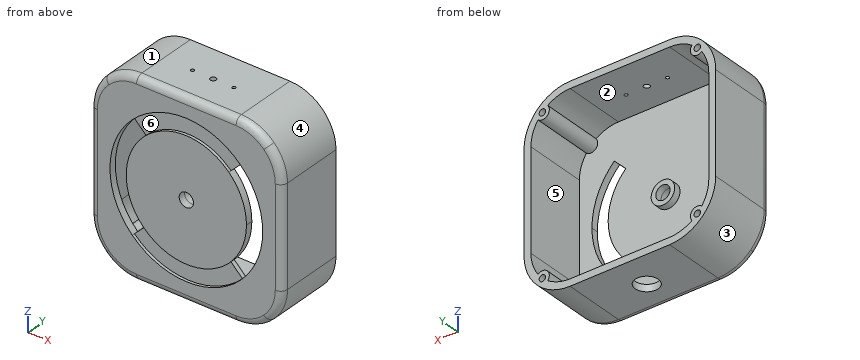
from build123d import *
from build123d.topology import SkipClean

# Parameters (mm, degrees)
SKETCH1_W           = 83.2
SKETCH1_H           = 83.2
BOSS_EXTRUDE1_DEPTH = 30
FILLET1_R           = 20
SHELL2_T            = -3
SKETCH2_R           = 1.25
SKETCH2_R_2         = 0.75
CUT_EXTRUDE1_DEPTH  = 30
SKETCH3_R           = 5
CUT_EXTRUDE2_DEPTH  = 30
SKETCH4_R           = 3.1
CUT_EXTRUDE3_DEPTH  = 30
CUT_EXTRUDE4_DEPTH  = 1.2
SKETCH6_R           = 5.1
SKETCH6_R_2         = 3.1
BOSS_EXTRUDE2_DEPTH = 3
SKETCH7_R           = 3
BOSS_EXTRUDE3_DEPTH = 27
SKETCH9_R           = 1.4
CUT_EXTRUDE5_DEPTH  = 27
FILLET2_R           = 3


with BuildPart() as part:
    # Sketch1 → Boss-Extrude1 (new body)
    with BuildSketch(Plane(origin=(0, 0, 0), x_dir=(1, 0, 0), z_dir=(0, 1, 0))):
        with Locations((-19.461988304, -3.284210526)):
            Rectangle(SKETCH1_W, SKETCH1_H)
    extrude(amount=BOSS_EXTRUDE1_DEPTH)

    # Fillet1
    fillet1_edges = [part.edges().sort_by_distance(p)[0] for p in [
        (-61.061988304, 15, -38.315789474),
        (22.138011696, 15, -38.315789474),
        (22.138011696, 15, 44.884210526),
        (-61.061988304, 15, 44.884210526),
    ]]
    fillet(fillet1_edges, radius=FILLET1_R)

    # Shell2
    shell2_openings = [part.faces().sort_by_distance(p)[0] for p in [
        (-19.461988304, 30, 3.284210526),
    ]]
    offset(amount=SHELL2_T, openings=shell2_openings, kind=Kind.INTERSECTION)

    # Sketch2 → Cut-Extrude1 (cut)
    with BuildSketch(Plane.XY.offset(44.884210526)):
        with Locations((-19.461988304, 15)):
            Circle(SKETCH2_R)
        with Locations((-10.461988304, 15)):
            Circle(SKETCH2_R_2)
        with Locations((-28.461988304, 15)):
            Circle(SKETCH2_R_2)
    extrude(amount=-CUT_EXTRUDE1_DEPTH, mode=Mode.SUBTRACT)

    # Sketch3 → Cut-Extrude2 (cut)
    with BuildSketch(Plane(origin=(0, 0, -38.315789474), x_dir=(-1, 0, 0), z_dir=(0, 0, -1))):
        with Locations((19.461988304, 15)):
            Circle(SKETCH3_R)
    extrude(amount=-CUT_EXTRUDE2_DEPTH, mode=Mode.SUBTRACT)

    # Sketch4 → Cut-Extrude3 (cut)
    with BuildSketch(Plane.XZ):
        with BuildLine():
            ThreePointArc((13.688011696, 3.284210526), (11.164618199, 15.970166309), (3.978601492, 26.724800323))
            Line((3.978601492, 26.724800323), (-1.006501315, 21.739697515))
            ThreePointArc((-1.006501315, 21.739697515), (4.651267494, 13.272248111), (6.638011696, 3.284210526))
            ThreePointArc((6.638011696, 3.284210526), (4.651267494, -6.703827058), (-1.006501315, -15.171276463))
            Line((-1.006501315, -15.171276463), (3.978601492, -20.15637927))
            ThreePointArc((3.978601492, -20.15637927), (11.164618199, -9.401745257), (13.688011696, 3.284210526))
        make_face()
        with BuildLine():
            Line((-37.917475293, 21.739697515), (-42.9025781, 26.724800323))
            ThreePointArc((-42.9025781, 26.724800323), (-52.611988304, 3.284210526), (-42.9025781, -20.15637927))
            Line((-42.9025781, -20.15637927), (-37.917475293, -15.171276463))
            ThreePointArc((-37.917475293, -15.171276463), (-45.561988304, 3.284210526), (-37.917475293, 21.739697515))
        make_face()
        with Locations(Location((-19.461988304, 3.284210526, 0), (0, 0, 270))):
            Circle(SKETCH4_R)
    extrude(amount=-CUT_EXTRUDE3_DEPTH, mode=Mode.SUBTRACT)

    # Sketch5 → Cut-Extrude4 (cut)
    with SkipClean():  # the faces are left unmerged after this step: merging them gives an invalid solid
        with BuildSketch(Plane.XZ):
            with BuildLine():
                Line((-42.9025781, 26.724800323), (-37.917475293, 21.739697515))
                ThreePointArc((-37.917475293, 21.739697515), (-19.461988304, 29.384210526), (-1.006501315, 21.739697515))
                Line((-1.006501315, 21.739697515), (3.978601492, 26.724800323))
                ThreePointArc((3.978601492, 26.724800323), (-19.461988304, 36.434210526), (-42.9025781, 26.724800323))
            make_face()
            with BuildLine():
                Line((-1.006501315, -15.171276463), (3.978601492, -20.15637927))
                ThreePointArc((3.978601492, -20.15637927), (-19.461988304, -29.865789474), (-42.9025781, -20.15637927))
                Line((-42.9025781, -20.15637927), (-37.917475293, -15.171276463))
                ThreePointArc((-37.917475293, -15.171276463), (-19.461988304, -22.815789474), (-1.006501315, -15.171276463))
            make_face()
        extrude(amount=-CUT_EXTRUDE4_DEPTH, mode=Mode.SUBTRACT)

    # Sketch6 → Boss-Extrude2 (add)
    with SkipClean():  # the faces are left unmerged after this step: merging them gives an invalid solid
        with BuildSketch(Plane(origin=(0, 3, 0), x_dir=(1, 0, 0), z_dir=(0, 1, 0))):
            with Locations(Location((-19.461988304, -3.284210526, 0), (0, 0, 270))):
                Circle(SKETCH6_R)
            with Locations(Location((-19.461988304, -3.284210526, 0), (0, 0, 90))):
                Circle(SKETCH6_R_2, mode=Mode.SUBTRACT)
        extrude(amount=BOSS_EXTRUDE2_DEPTH)

    # Sketch7 → Boss-Extrude3 (add)
    with SkipClean():  # the faces are left unmerged after this step: merging them gives an invalid solid
        with BuildSketch(Plane(origin=(0, 3, 0), x_dir=(1, 0, 0), z_dir=(0, 1, 0))):
            with Locations((-53.082803584, 30.336604754)):
                Circle(SKETCH7_R)
            with Locations((-53.082803584, -36.905025806)):
                Circle(SKETCH7_R)
            with Locations((14.158826976, -36.905025806)):
                Circle(SKETCH7_R)
            with Locations((14.158826976, 30.336604754)):
                Circle(SKETCH7_R)
        extrude(amount=BOSS_EXTRUDE3_DEPTH)

    # Sketch9 → Cut-Extrude5 (cut)
    with SkipClean():  # the faces are left unmerged after this step: merging them gives an invalid solid
        with BuildSketch(Plane(origin=(0, 30, 0), x_dir=(1, 0, 0), z_dir=(0, 1, 0))):
            with Locations(Location((-53.082803584, 30.336604754, 0), (0, 0, 270))):
                Circle(SKETCH9_R)
            with Locations(Location((14.158826976, 30.336604754, 0), (0, 0, 270))):
                Circle(SKETCH9_R)
            with Locations(Location((14.158826976, -36.905025806, 0), (0, 0, 270))):
                Circle(SKETCH9_R)
            with Locations(Location((-53.082803584, -36.905025806, 0), (0, 0, 270))):
                Circle(SKETCH9_R)
        extrude(amount=-CUT_EXTRUDE5_DEPTH, mode=Mode.SUBTRACT)

    # Fillet2
    fillet2_edges = [part.edges().sort_by_distance(p)[0] for p in [
        (22.138011696, 0, 3.284210526),
        (-61.061988304, 0, 3.284210526),
        (-19.461988304, 0, -38.315789474),
        (-19.461988304, 0, 44.884210526),
        (-55.204123928, 0, 39.02634615),
        (-55.204123928, 0, -32.457925097),
        (16.28014732, 0, -32.457925097),
        (16.28014732, 0, 39.02634615),
    ]]
    fillet(fillet2_edges, radius=FILLET2_R)


solid = part.part
For this review, take the finished solid that the model builds, in its own axes (mm). Face numbers are marked on the shaded views. A direction names the side the tool comes from. Round coordinates to 2 decimals unless told otherwise and drop trailing zeros. Loops run counter-clockwise (first coordinate to the right, second up) from the corner with the lowest first, then second, coordinate; pieces in that order, holes last. Notation, with made-up numbers: (61.5, 0.25) - (84.5, 0.25) arc R20 ccw to (84.5, 37.25) - close; hole circle Ø7 at (51.25, 65.5). An arc over 180 degrees is marked (long way). Put each result on its own line as item: value. Start each with the question number.
1. Consider section D-D on x = -39.5. State the section outline as (y, z) points, plus the area to 3 significant figures.
2. Insertion check: P1, Ø2, axis at x = -11.5, z = -23.5, coming from the +Y side; P2, Ø8, axis at y = 14.5, z = 36.5, coming from the +X side; P3, Ø1.5, axis at y = 11.5, z = -28.5, coming from the -X side. Each pin has a flat end and moves straight along its axis. Give the tip position at first contact, or say it passes through.
3. For probe 1 along Z at (x, y) = (-27.5, 10); probe 2 along X at (y, z) = (6, 21); probe 3 along Z at (x, y) = (15, 11), list the stretches that pass through material, from the lowest coordinate up. Write a range as [from, to].
4. Consider section B-B on x = 0. State the section outline as (y, z) points.
5. Consider section C-C on y = 12.5. State how many separate pieces and enclosed holes the cut face has, plus the area to 3 significant figures.
6. Consider section A-A on z = 15. State the section outline as (x, y) points.
7. Mouldability with a two-part tool opening along Z and no side actions: class the marked faces 1, 2 and 3 as +Z half, -Z half, draft (parallel to the pull), parting line (faces both ways), or undercut.
8. For the marked faces 4, 5 and 6, list the 3-axis set-ups (+Z, -Z, +X, -X, +Y, -Y) from which the entire face can be reached by the end or side of a thin tool; tool diameter is ignored.
Result sheet:
1. outline: (0, -35.32) arc R3 ccw to (3, -38.32) - (30, -38.32) - (30, -35.32) - (3, -35.32) - (3, -16.75) - (1.2, -16.75) - (1.2, -23.12) - (0, -23.12) - close; (0, -13.44) - (3, -13.44) - (3, 20.01) - (0, 20.01) - close; (0, 29.69) - (1.2, 29.69) - (1.2, 23.32) - (3, 23.32) - (3, 41.88) - (30, 41.88) - (30, 44.88) - (3, 44.88) arc R3 ccw to (0, 41.88) - close
1. area: 373 mm^2
2. P1: y = 3
2. P2: x = 20.63
2. P3: x = -58.7
3. probe 1: [-38.32, -35.32], [41.88, 44.88]
3. probe 2: [-61.06, -58.06], [19.14, 22.14]
3. probe 3: [-33.63, -31.46], [-29.22, -27.46], [34.03, 35.79], [38.02, 40.2]
4. outline: (0, -35.32) arc R3 ccw to (3, -38.32) - (30, -38.32) - (30, -35.32) - (3, -35.32) - (3, -16.18) - (1.2, -16.18) - (1.2, -23.55) - (0, -23.55) - close; (0, -14.11) - (3, -14.11) - (3, 20.68) - (0, 20.68) - close; (0, 30.12) - (1.2, 30.12) - (1.2, 22.75) - (3, 22.75) - (3, 41.88) - (30, 41.88) - (30, 44.88) - (3, 44.88) arc R3 ccw to (0, 41.88) - close
5. separate pieces: 1
5. enclosed holes: 4
5. area: 871 mm^2
6. outline: (-61.06, 3) arc R3 ccw to (-58.06, 0) - (-50.47, 0) - (-50.47, 3) - (-58.06, 3) - (-58.06, 30) - (-61.06, 30) - close; (-42.78, 0) - (3.86, 0) - (3.86, 3) - (-42.78, 3) - close; (11.55, 0) - (19.14, 0) arc R3 ccw to (22.14, 3) - (22.14, 30) - (19.14, 30) - (19.14, 3) - (11.55, 3) - close
7. face 1: +Z half
7. face 2: undercut
7. face 3: -Z half
8. face 4: +Z, +X, +Y, -Y
8. face 5: +Y
8. face 6: -Y
